Study the drawing (mm; zero at the part's minimum x, y, z) and answer. Give positions to 0.01 mm unless a question says otherwise; leave off trailing zeros. Order: outer loops, then holes, each group sorted by start corner. A loop starts at its lowest first (then second) coordinate and runs counter-clockwise, first axis right, second up. Notation, with made-up numbers: (80.5, 37.5) - (122.5, 37.5) arc R15 cw to (122.5, 63.5) - close; hole circle Ø1 at (14, 34.25). An arc over 180 degrees is marked (long way). Put each result on its own line as item: value.
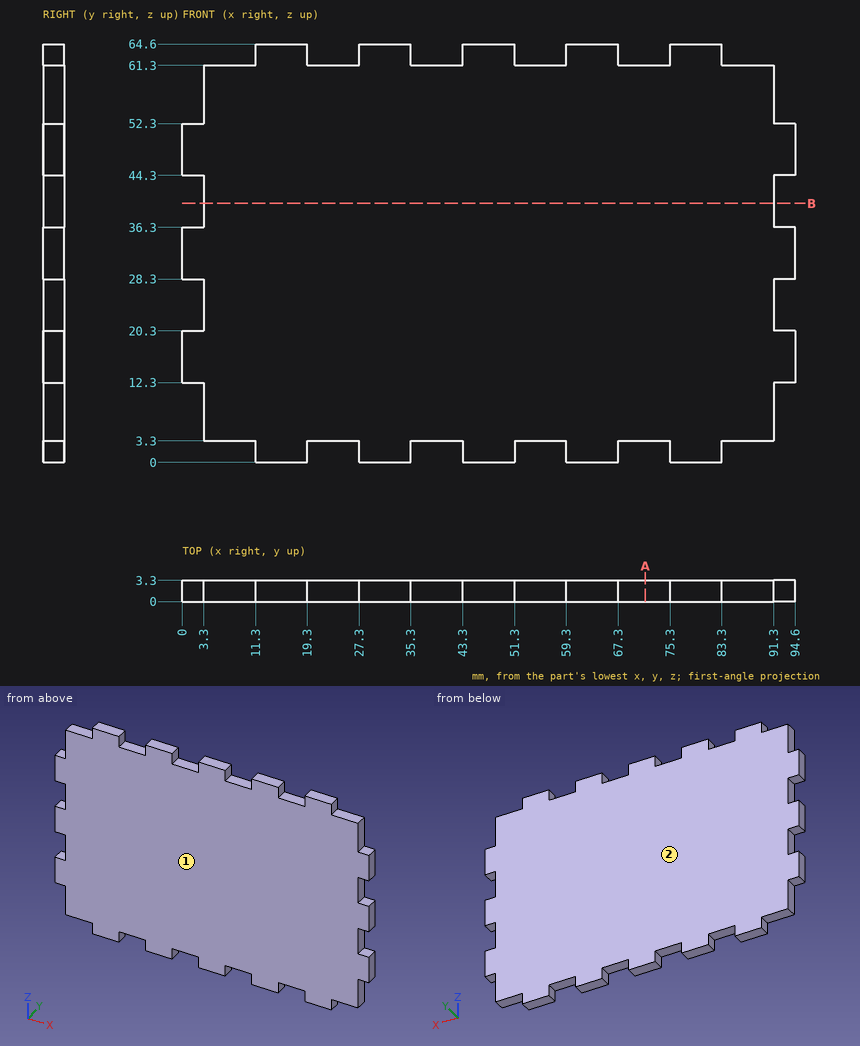
(1) Section B-B, the plane z = 40 is taken. Write down the section's boundary in (x, y), then the cut area to 3 significant figures.
Geometry check:
outline: (3.3, 0) - (91.3, 0) - (91.3, 3.3) - (3.3, 3.3) - close
area: 290 mm²
(2) Straight lines are drawn through the part: line 1 (X direction, y = 2.65, z = 25); line 2 (Z direction, x = 40.5, y = 0.85). For each, find the intervals that lie inside material, in ascending order.
Geometry check:
line 1: x = 3.3 to 91.3
line 2: z = 3.3 to 61.3
(3) Section A-A, the plane x = 71.5 is taken. Write down the section's boundary in (y, z).
Geometry check:
outline: (0, 3.3) - (3.3, 3.3) - (3.3, 61.3) - (0, 61.3) - close
(4) Determine the mould class of the marked faces 1 and 2 for opening direction Y: pulls with the +Y half, pulls with the -Y half, needs draft (parallel to the pull), parting line crosses it, or undercut.
Geometry check:
face 1: pulls with the -Y half
face 2: pulls with the +Y half
(5) Given pin 1 (1.6 mm diameter, centred on x = 21.5, y = 2, fed in from +Z); pin 2 (1.6 mm diameter, centred on y = 1.5, z = 25, fed in from +X); pin 3 (1 mm diameter, centred on y = 1.5, z = 2.5, fed in from +X), each flat-ended and moving along its own axis, determine where each tip first touches the part or whether it passes through.
Geometry check:
pin 1: stops at z = 61.3
pin 2: stops at x = 91.3
pin 3: stops at x = 83.3
